Verification items for the finished model (mm, model axes). A direction names the side the tool comes from. Coordinates: 2 decimals unless noted, no trailing zeros. Order: outer loops, then holes, each group sorted by start corner. A loop starts at its lowest first (then second) coordinate and runs counter-clockwise, first axis right, second up. Notation, with made-up numbers: M 75,72.5 L 91,72.5 A22 ccw 91,83.5 Z; hole C 71,89 d10. An arc over 180 degrees is marked long. Write item = value, one per line.
```python
from build123d import *

# Parameters (mm, degrees)
SKETCH_1_R          = 1.52
EXTRUDE_1_DEPTH     = 7
SKETCH_2_R          = 1.52
SKETCH_2_R_2        = 1.520000001
CUT_EXTRUDE_2_DEPTH = 10
FILLET_1_R          = 8
FILLET_3_R          = 1
FILLET_4_R          = 5
FILLET_5_R          = 1.5
SKETCH_3_R          = 2.02
SKETCH_3_R_2        = 1.52
CUT_EXTRUDE_3_DEPTH = 10


with BuildPart() as part:
    # 草图1 → 凸台-拉伸1 (new body)
    with BuildSketch(Plane(origin=(0, 0, 0), x_dir=(1, 0, 0), z_dir=(0, 1, 0))):
        Polygon((12, -0.002444932), (12, 140.81), (30.355391701, 140.81), (30.355391701, 181.996219272), (-18.063025957, 181.996219272), (-18.063025957, 140.81), (0, 140.81), (0, -0.002444932), (-9.306341863, -0.002444932), (-9.306341863, -16.766517892), (21.308530359, -16.766517892), (21.308530359, -0.002444932), align=None)
        with Locations((6, 24.810293178)):
            Circle(SKETCH_1_R, mode=Mode.SUBTRACT)
    extrude(amount=EXTRUDE_1_DEPTH)

    # 草图2 → 切除-拉伸2 (cut)
    with BuildSketch(Plane(origin=(0, 7, 0), x_dir=(1, 0, 0), z_dir=(0, 1, 0))):
        with BuildLine():
            ThreePointArc((9.6, 155.810000018), (3.454415588, 158.35558443), (6, 152.210000018))
            Line((6, 152.210000018), (6, 155.810000018))
            Line((6, 155.810000018), (9.6, 155.810000018))
        make_face()
        with BuildLine():
            Line((6, 155.810000018), (6, 152.210000018))
            ThreePointArc((6, 152.210000018), (7.377660354, 152.4840337), (8.545584409, 153.264415603))
            Line((8.545584409, 153.264415603), (6, 155.810000018))
        make_face()
        with BuildLine():
            Line((9.6, 155.810000018), (6, 155.810000018))
            Line((6, 155.810000018), (8.545584409, 153.264415603))
            ThreePointArc((8.545584409, 153.264415603), (9.325966316, 154.43233966), (9.6, 155.810000018))
        make_face()
        with Locations((-0.748108245, 148.915708883)):
            Circle(SKETCH_2_R)
        with Locations((0.666105318, 150.329922446)):
            Circle(SKETCH_2_R)
        with BuildLine():
            Line((-0.40869699, 151.404724753), (-1.822910552, 149.990511191))
            ThreePointArc((-1.822910552, 149.990511191), (-1.376757591, 150.299616395), (-0.850445717, 150.432259918))
            ThreePointArc((-0.850445717, 150.432259918), (-0.717802194, 150.958571792), (-0.40869699, 151.404724753))
        make_face()
        with BuildLine():
            ThreePointArc((0.76844279, 148.813371411), (0.635799267, 148.287059538), (0.326694063, 147.840906576))
            Line((0.326694063, 147.840906576), (1.740907625, 149.255120138))
            ThreePointArc((1.740907625, 149.255120138), (1.294754663, 148.946014934), (0.76844279, 148.813371411))
        make_face()
        with BuildLine():
            Line((10.405275239, 149.255120151), (11.819488799, 147.840906587))
            ThreePointArc((11.819488799, 147.840906586), (11.510383595, 148.287059549), (11.377740072, 148.813371422))
            ThreePointArc((11.377740072, 148.813371422), (10.851428199, 148.946014947), (10.405275239, 149.255120151))
        make_face()
        with BuildLine():
            Line((11.480077548, 150.329922457), (10.405275241, 151.404724766))
            ThreePointArc((10.405275241, 151.404724766), (9.960077548, 150.329922459), (10.405275239, 149.255120151))
            ThreePointArc((10.405275239, 149.255120151), (10.851428199, 148.946014947), (11.377740072, 148.813371422))
            ThreePointArc((11.377740072, 148.813371422), (11.471198506, 149.449757066), (11.819488801, 149.990511203))
            Line((11.819488801, 149.990511203), (11.480077548, 150.329922457))
        make_face()
        with BuildLine():
            Line((12.554879856, 151.404724763), (11.480077548, 150.329922457))
            Line((11.480077548, 150.329922457), (11.819488801, 149.990511203))
            ThreePointArc((11.819488801, 149.990511203), (12.360242939, 150.338801496), (12.996628583, 150.432259929))
            ThreePointArc((12.996628583, 150.432259929), (12.863985059, 150.958571802), (12.554879856, 151.404724763))
        make_face()
        with BuildLine():
            Line((11.819488801, 149.990511203), (12.554879854, 149.255120148))
            ThreePointArc((12.554879854, 149.255120148), (12.884374437, 149.748243639), (13.000077548, 150.329922457))
            ThreePointArc((13.000077548, 150.329922457), (12.999215062, 150.381120244), (12.996628583, 150.432259929))
            ThreePointArc((12.996628583, 150.432259929), (12.360242939, 150.338801496), (11.819488801, 149.990511203))
        make_face()
        with BuildLine():
            ThreePointArc((11.377740072, 148.813371422), (12.014125716, 148.906829855), (12.554879854, 149.255120148))
            Line((12.554879854, 149.255120148), (11.819488801, 149.990511203))
            ThreePointArc((11.819488801, 149.990511203), (11.471198506, 149.449757066), (11.377740072, 148.813371422))
        make_face()
        with BuildLine():
            ThreePointArc((12.554879856, 151.404724763), (11.480077549, 151.849922457), (10.405275241, 151.404724766))
            Line((10.405275241, 151.404724766), (11.480077548, 150.329922457))
            Line((11.480077548, 150.329922457), (12.554879856, 151.404724763))
        make_face()
        with BuildLine():
            Line((13.969093417, 149.990511199), (12.554879856, 151.404724763))
            ThreePointArc((12.554879856, 151.404724763), (12.863985059, 150.958571802), (12.996628583, 150.432259929))
            ThreePointArc((12.996628583, 150.432259929), (13.522940456, 150.299616405), (13.969093418, 149.9905112))
        make_face()
        with BuildLine():
            Line((12.554879854, 149.255120148), (12.894291108, 148.915708893))
            Line((12.894291108, 148.915708893), (13.969093417, 149.990511199))
            ThreePointArc((13.969093418, 149.9905112), (13.522940456, 150.299616405), (12.996628583, 150.432259929))
            ThreePointArc((12.996628583, 150.432259929), (12.999215062, 150.381120244), (13.000077548, 150.329922457))
            ThreePointArc((13.000077548, 150.329922457), (12.884374437, 149.748243639), (12.554879854, 149.255120148))
        make_face()
        with BuildLine():
            Line((12.894291108, 148.915708893), (13.969093415, 147.840906584))
            ThreePointArc((13.969093415, 147.840906584), (14.298587998, 148.334030075), (14.414291109, 148.915708893))
            ThreePointArc((14.414291109, 148.915708893), (14.298587999, 149.49738771), (13.969093418, 149.9905112))
            Line((13.969093417, 149.990511199), (12.894291108, 148.915708893))
        make_face()
        with Locations((11.480077548, 161.290077579)):
            Circle(SKETCH_2_R)
        with Locations((12.894291108, 162.704291143)):
            Circle(SKETCH_2_R_2)
        with BuildLine():
            ThreePointArc((11.377740072, 162.806628614), (11.510383595, 163.332940488), (11.819488799, 163.77909345))
            Line((11.819488799, 163.779093449), (10.405275239, 162.364879885))
            ThreePointArc((10.405275239, 162.364879885), (10.851428199, 162.673985089), (11.377740072, 162.806628614))
        make_face()
        with BuildLine():
            ThreePointArc((12.996628583, 161.187740107), (12.863985059, 160.661428234), (12.554879856, 160.215275273))
            Line((12.554879856, 160.215275273), (13.969093417, 161.629488837))
            ThreePointArc((13.969093418, 161.629488836), (13.522940456, 161.320383631), (12.996628583, 161.187740107))
        make_face()
        with Locations((0.666105329, 161.290077566)):
            Circle(SKETCH_2_R)
        with Locations((-0.74810823, 162.704291131)):
            Circle(SKETCH_2_R)
        with BuildLine():
            Line((1.740907642, 162.364879874), (0.326694079, 163.779093436))
            ThreePointArc((0.326694079, 163.779093436), (0.635799282, 163.332940474), (0.768442805, 162.8066286))
            ThreePointArc((0.768442805, 162.8066286), (1.294754678, 162.673985076), (1.740907639, 162.364879871))
        make_face()
        with BuildLine():
            ThreePointArc((-0.850445706, 161.187740096), (-1.376757579, 161.320383621), (-1.82291054, 161.629488826))
            Line((-1.82291054, 161.629488826), (-0.408696978, 160.215275263))
            ThreePointArc((-0.408696981, 160.21527526), (-0.717802184, 160.661428223), (-0.850445706, 161.187740096))
        make_face()
        Polygon((-18.063025957, 181.996219272), (-18.063025957, 140.81), (-2.660254048, 140.81), (-11.320508097, 155.810000018), (-2.660254048, 170.810000036), (14.660254048, 170.810000036), (23.320508097, 155.810000018), (16.980762117, 144.829237874), (14.660254048, 140.81), (30.355391701, 140.81), (30.355391701, 181.996219272), align=None)
        with BuildLine():
            ThreePointArc((11.819488799, 147.840906586), (12.894291106, 147.395708892), (13.969093415, 147.840906584))
            Line((13.969093415, 147.840906584), (12.894291108, 148.915708893))
            Line((12.894291108, 148.915708893), (12.554879854, 149.255120148))
            ThreePointArc((12.554879854, 149.255120148), (12.014125716, 148.906829855), (11.377740072, 148.813371422))
            ThreePointArc((11.377740072, 148.813371422), (11.510383595, 148.287059549), (11.819488799, 147.840906586))
        make_face()
    extrude(amount=-CUT_EXTRUDE_2_DEPTH, mode=Mode.SUBTRACT)

    # 圆角1
    fillet_1_edges = [part.edges().sort_by_distance(p)[0] for p in [
        (0, 3.5, 0.002444932),
        (12, 3.5, 0.002444932),
    ]]
    fillet(fillet_1_edges, radius=FILLET_1_R)

    # 圆角3
    fillet_3_edges = [part.edges().sort_by_distance(p)[0] for p in [
        (-9.306341863, 3.5, 0.002444932),
        (21.308530359, 3.5, 0.002444932),
    ]]
    fillet(fillet_3_edges, radius=FILLET_3_R)

    # 圆角4
    fillet_4_edges = [part.edges().sort_by_distance(p)[0] for p in [
        (21.308530359, 3.5, 16.766517892),
        (-9.306341863, 3.5, 16.766517892),
    ]]
    fillet(fillet_4_edges, radius=FILLET_4_R)

    # 圆角5
    fillet_5_edges = [part.edges().sort_by_distance(p)[0] for p in [
        (0, 3.5, -140.81),
        (12, 3.5, -140.81),
        (-11.320508097, 3.5, -155.810000018),
        (-2.660254048, 3.5, -140.81),
        (14.660254048, 3.5, -140.81),
        (23.320508097, 3.5, -155.810000018),
        (14.660254048, 3.5, -170.810000036),
        (-2.660254048, 3.5, -170.810000036),
    ]]
    fillet(fillet_5_edges, radius=FILLET_5_R)

    # 草图3 → 切除-拉伸3 (cut)
    with BuildSketch(Plane(origin=(0, 0, 0), x_dir=(-1, 0, 0), z_dir=(0, -1, 0))):
        with Locations((-17.66726189, -2.022444932)):
            Circle(SKETCH_3_R)
        with Locations((5.66726189, -2.022444932)):
            Circle(SKETCH_3_R)
        with Locations((-6, -13.689706822)):
            Circle(SKETCH_3_R_2)
    extrude(amount=-CUT_EXTRUDE_3_DEPTH, mode=Mode.SUBTRACT)


solid = part.part
```
Item 1: Sectioned sample at B-B, the plane y = 2.25. Give the number of separate pieces and of enclosed holes in the cut face, then the cut area to 3 significant figures.
Report:
separate_pieces = 1
enclosed_holes = 9
area = 2,860 mm^2
Item 2: Release check for a two-part mould opening along X. For faces 1 (the cylindrical face through (-7.803, 3.549, 15.341)), 2 (the cylindrical face through (5.67, 3.451, -23.326)), 3 (the cylindrical face through (14.281, 3.549, -2.403)) record: pulls with the +X half, pulls with the -X half, needs draft (parallel to the pull), parting line crosses it, or undercut.
Report:
face_1 = pulls with the -X half
face_2 = undercut
face_3 = pulls with the +X half
Item 3: Gauge pin test, flat ends, axial feed: pin 1 (1.8 mm diameter, centred on x = 6, z = 13.69, fed in from -Y); pin 2 (3 mm diameter, centred on y = 5, z = -53, fed in from -X); pin 3 (1.5 mm diameter, centred on y = 3.5, z = -108, fed in from +X); pin 4 (3.5 mm diameter, centred on y = 4, z = 8.5, fed in from -X). Record the tip position at first contact, or that the pin passes through.
Report:
pin_1 = through
pin_2 = 0
pin_3 = 12
pin_4 = -9.31
Item 4: Tool access check on faces 4 (the cylindrical face through (6.33, 3.451, 15.174)), 5 (the flat face through (12, 3, -73)), 6 (the flat face through (21.309, 3, 6)), 7 (the cylindrical face through (-2.406, 3.549, -2.279)), 8 (the flat face through (-9.306, 3, 6)). Record the directions out of +Z, -Z, +X, -X, +Y, -Y that give a thin tool (end or side, any length) a straight path to the whole face; none if there is none.
Report:
face_4 = +Y, -Y
face_5 = +X, +Y, -Y
face_6 = +Z, +X, +Y, -Y
face_7 = -X, +Y, -Y
face_8 = +Z, -X, +Y, -Y
Item 5: Sectioned sample at A-A, the plane z = -39. Enter the section's corners in (x, y).
Report:
outline = M 0,0 L 12,0 L 12,7 L 0,7 Z
Item 6: Scan lines: L1, parallel to Z at x = 6, y = 2.5; L2, parallel to Z at x = 11, y = 2.5; L3, parallel to Z at x = 5.5, y = 1.25. Record each from-to range of solid material in increasing order. Write a range as from..to.
Report:
L1 = -170.81..-159.41, -152.21..-26.33, -23.29..12.17, 15.21..16.77
L2 = -170.81..-162.96, -159.85..-151.77, -148.66..16.77
L3 = -170.81..-159.38, -152.24..-26.25, -23.37..12.25, 15.13..16.77
